from build123d import *

# Parameters (mm, degrees)
SKETCH_1_W          = 108
SKETCH_1_H          = 65
SKETCH_1_W_2        = 99
SKETCH_1_H_2        = 42
EXTRUDE_1_DEPTH     = 5
SKETCH_2_W          = 108
SKETCH_2_H          = 65
SKETCH_2_W_2        = 100
SKETCH_2_H_2        = 62
SKETCH_2_W_3        = 7
SKETCH_2_H_3        = 7
EXTRUDE_2_DEPTH     = 5
SKETCH_3_W          = 108
SKETCH_3_H          = 65
EXTRUDE_4_DEPTH     = 3
SKETCH_4_R          = 1.15
CUT_EXTRUDE_1_DEPTH = 7


with BuildPart() as part:
    # 草圖1 → 填料-伸長1 (new body)
    with BuildSketch(Plane.XY):
        with Locations((10.575206568, -6.470178926)):
            Rectangle(SKETCH_1_W, SKETCH_1_H)
        with Locations((10.575206568, -6.470178926)):
            Rectangle(SKETCH_1_W_2, SKETCH_1_H_2, mode=Mode.SUBTRACT)
    extrude(amount=EXTRUDE_1_DEPTH)

    # 草圖2 → 填料-伸長2 (add)
    # profile 1 of 5: a face of its own
    with BuildSketch(Plane.XY.offset(5)):
        with Locations((10.575206568, -6.470178926)):
            Rectangle(SKETCH_2_W, SKETCH_2_H)
        with Locations((10.575206568, -6.470178926)):
            Rectangle(SKETCH_2_W_2, SKETCH_2_H_2, mode=Mode.SUBTRACT)
    # profile 2 of 5: a face of its own
    with BuildSketch(Plane.XY.offset(5)):
        with Locations((-35.924793432, 21.029821074)):
            Rectangle(SKETCH_2_W_3, SKETCH_2_H_3)
    # profile 3 of 5: a face of its own
    with BuildSketch(Plane.XY.offset(5)):
        with Locations((57.075206568, 21.029821074)):
            Rectangle(SKETCH_2_W_3, SKETCH_2_H_3)
    # profile 4 of 5: a face of its own
    with BuildSketch(Plane.XY.offset(5)):
        with Locations((57.075206568, -33.970178926)):
            Rectangle(SKETCH_2_W_3, SKETCH_2_H_3)
    # profile 5 of 5: a face of its own
    with BuildSketch(Plane.XY.offset(5)):
        with Locations((-35.924793432, -33.970178926)):
            Rectangle(SKETCH_2_W_3, SKETCH_2_H_3)
    extrude(amount=EXTRUDE_2_DEPTH)

    # 草圖3 → 填料-伸長4 (add)
    with BuildSketch(Plane.XY.offset(10)):
        with Locations((10.575206568, -6.470178926)):
            Rectangle(SKETCH_3_W, SKETCH_3_H)
        Polygon((-39.424793432, -37.470178926), (-32.424793432, -37.470178926), (53.575206568, -37.470178926), (60.575206568, -37.470178926), (60.575206568, -30.470178926), (60.575206568, 17.529821074), (60.575206568, 24.529821074), (53.575206568, 24.529821074), (-32.424793432, 24.529821074), (-39.424793432, 24.529821074), (-39.424793432, 17.529821074), (-39.424793432, -30.470178926), align=None, mode=Mode.SUBTRACT)
    extrude(amount=EXTRUDE_4_DEPTH)

    # 草圖4 → 除料-伸長1 (cut)
    with BuildSketch(Plane.XY.offset(10)):
        with Locations((-35.924793432, 21.029821074)):
            Circle(SKETCH_4_R)
        with Locations((57.075206568, 21.029821074)):
            Circle(SKETCH_4_R)
        with Locations((57.075206568, -33.970178926)):
            Circle(SKETCH_4_R)
        with Locations((-35.924793432, -33.970178926)):
            Circle(SKETCH_4_R)
    extrude(amount=-CUT_EXTRUDE_1_DEPTH, mode=Mode.SUBTRACT)


solid = part.part
Source: CAD feature listing. Evaluate the final solid. Frame: model axes, mm. A direction names the side the tool comes from. Give positions to 0.01 mm unless a question says otherwise; leave off trailing zeros. Write each loop counter-clockwise with the first axis right and the second up, starting at its lowest first coordinate (ties: lowest second). Pieces come first, ordered by that corner, then holes. Notation, with made-up numbers: (6.25, -34.75) -> (49.25, -34.75) arc R23 ccw to (49.25, -5.75) -> close; hole circle Ø3 at (48, 67.25). An arc over 180 degrees is marked (long way). Return JSON: item names as keys, results as strings. Group by question number.
1. Section C-C, the plane y = -21.5. Output: boundary loops of the cut face in (x, z), then the cut area to 3 significant figures.
2. Section B-B, the plane z = 1.5. Output: boundary loops of the cut face in (x, y).
3. Section D-D, the plane z = 7.75. Output: boundary loops of the cut face in (x, y).
4. Access query for faces 3 (the face through (53.575, -34, 7)), 4 (the face through (-38.925, -7, 2)), 5 (the face through (64.575, -7, 6)). Directions: +Z, -Z, +X, -X, +Y, -Y. A direction counts if a zero-diameter tool reaches every point of the face in a straight line with its end or side. Return the directions, or none.
5. Mould query, pull axis Y, two halves, no side actions, for faces 1 (the face through (-43.425, -7, 6)), 2 (the face through (10, 14.53, 2)). Classes: +Y half, -Y half, draft (parallel to the pull), parting line (faces both ways), or undercut.
6. Pin query (flat end, axial travel): pin 1 Ø2.5 at (x, y) = (-35.92, 21.03) entering from +Z; pin 2 Ø1.1 at (x, y) = (-36, -34.5) entering from +Z; pin 3 Ø3 at (x, y) = (27.5, 16) entering from +Z. Return the tip coordinate at first contact, or that it passes through.
7. Material intervals for line 1 (X direction, y = -6.5, z = 10.75); line 2 (X direction, y = 1.5, z = 4.75); line 3 (Y direction, x = 2.5, z = 1.5), sorted ascending. Write a range as from..to.
8. Section A-A, the plane x = 28. Output: boundary loops of the cut face in (y, z), then the cut area to 3 significant figures.
Determined:
{
 "1": {"outline": "(-43.42, 0) -> (-38.92, 0) -> (-38.92, 5) -> (-39.42, 5) -> (-39.42, 13) -> (-43.42, 13) -> close; (60.08, 0) -> (64.58, 0) -> (64.58, 13) -> (60.58, 13) -> (60.58, 5) -> (60.08, 5) -> close", "area": "109 mm2"},
 "2": {"outline": "(-43.42, -38.97) -> (64.58, -38.97) -> (64.58, 26.03) -> (-43.42, 26.03) -> close; hole (-38.92, -27.47) -> (60.08, -27.47) -> (60.08, 14.53) -> (-38.92, 14.53) -> close"},
 "3": {"outline": "(-43.42, -38.97) -> (64.58, -38.97) -> (64.58, 26.03) -> (-43.42, 26.03) -> close; hole (-39.42, -30.47) -> (-32.42, -30.47) -> (-32.42, -37.47) -> (53.58, -37.47) -> (53.58, -30.47) -> (60.58, -30.47) -> (60.58, 17.53) -> (53.58, 17.53) -> (53.58, 24.53) -> (-32.42, 24.53) -> (-32.42, 17.53) -> (-39.42, 17.53) -> close; hole circle Ø2.3 at (-35.92, -33.97); hole circle Ø2.3 at (-35.92, 21.03); hole circle Ø2.3 at (57.08, -33.97); hole circle Ø2.3 at (57.08, 21.03)"},
 "4": {"face 3": "+Z", "face 4": "+Z, -Z", "face 5": "+Z, -Z, +X, +Y, -Y"},
 "5": {"face 1": "draft", "face 2": "undercut"},
 "6": {"pin 1": "stops at z = 10", "pin 2": "stops at z = 3", "pin 3": "stops at z = 5"},
 "7": {"line 1": "x = -43.42..-39.42, 60.58..64.58", "line 2": "x = -43.42..-38.92, 60.08..64.58", "line 3": "y = -38.97..-27.47, 14.53..26.03"},
 "8": {"outline": "(-38.97, 0) -> (-27.47, 0) -> (-27.47, 5) -> (-37.47, 5) -> (-37.47, 13) -> (-38.97, 13) -> close; (14.53, 0) -> (26.03, 0) -> (26.03, 13) -> (24.53, 13) -> (24.53, 5) -> (14.53, 5) -> close", "area": "139 mm2"}
}
